from build123d import *

# Parameters (mm, degrees)
BOSS_EXTRUDE1_DEPTH      = 31.75
BOSS_EXTRUDE1_DEPTH_BACK = 31.75
CUT_EXTRUDE2_DEPTH       = 76.011139841
SKETCH3_W                = 3.175
SKETCH3_H                = 76.2
CUT_EXTRUDE3_DEPTH       = 91.870466503


with BuildPart() as part:
    # Sketch1 → Boss-Extrude1 (new body, two sides)
    with BuildSketch(Plane(origin=(0, 0, 0), x_dir=(0, 0, -1), z_dir=(1, 0, 0))) as boss_extrude1_sk:
        with BuildLine():
            Line((1.021340573, 1065.671760022), (10.69404187, 1079.103015809))
            ThreePointArc((10.69404187, 1079.103015809), (11.573445276, 1080.842426323), (11.876332412, 1082.767824636))
            Line((11.876332412, 1082.767824636), (11.876332412, 1187.719530026))
            Line((11.876332412, 1187.719530026), (-13.536061703, 1215.286446683))
            Line((-13.536061703, 1215.286446683), (-19.823769094, 1336.738131825))
            Line((-19.823769094, 1336.738131825), (-36.668668575, 1336.738131825))
            Line((-36.668668575, 1336.738131825), (-41.611308298, 1332.181789519))
            Line((-41.611308298, 1332.181789519), (-19.823769313, 820.101609747))
            ThreePointArc((-19.823769313, 820.101609747), (-14.269049163, 657.404177816), (-11.609546724, 494.633675821))
            ThreePointArc((-11.609546724, 494.633675821), (-11.552697494, 390.848511752), (-12.926889154, 287.072430162))
            ThreePointArc((-12.926889154, 287.072430162), (-14.08497073, 249.282151425), (-16.036320575, 211.524522345))
            ThreePointArc((-16.036320575, 211.524522345), (-18.862629391, 134.694563635), (-17.789412377, 57.820128469))
            ThreePointArc((-17.789412377, 57.820128469), (-14.713555739, 31.224003963), (-7.655684583, 5.397637832))
            ThreePointArc((-7.655684583, 5.397637832), (0, 0), (7.655684583, 5.397637832))
            ThreePointArc((7.655684583, 5.397637832), (14.877278089, 28.754462777), (20.079353087, 52.642348827))
            ThreePointArc((20.079353087, 52.642348827), (27.352586181, 104.395526294), (31.292623673, 156.508551558))
            ThreePointArc((31.292623673, 156.508551558), (31.58109291, 163.474292498), (31.841795924, 170.441127883))
            ThreePointArc((31.841795924, 170.441127883), (33.322524829, 278.033900996), (30.144822487, 385.589931009))
            ThreePointArc((30.144822487, 385.589931009), (12.959303763, 715.76096893), (-4.76677265, 1045.903426895))
            ThreePointArc((-4.76677265, 1045.903426895), (-3.565814336, 1056.283327954), (1.021340573, 1065.671760022))
        make_face()
    extrude(amount=BOSS_EXTRUDE1_DEPTH)
    extrude(boss_extrude1_sk.sketch, amount=-BOSS_EXTRUDE1_DEPTH_BACK)

    # Sketch2 → Cut-Extrude2 (cut, through all)
    with BuildSketch(Plane.XY.offset(-33.399831543)):
        with BuildLine():
            Line((3.96875, 1336.738131825), (19.05, 293.18430056))
            ThreePointArc((19.05, 293.18430056), (18.724333894, 153.044911462), (13.698146022, 12.995306427))
            ThreePointArc((13.698146022, 12.995306427), (9.440831446, 3.765721828), (0, 0))
            Line((0, 0), (31.75, 0))
            Line((31.75, 0), (31.75, 1336.738131825))
            Line((31.75, 1336.738131825), (3.96875, 1336.738131825))
        make_face()
        with BuildLine():
            Line((-31.75, 0), (0, 0))
            ThreePointArc((0, 0), (-9.440831446, 3.765721828), (-13.698146022, 12.995306427))
            ThreePointArc((-13.698146022, 12.995306427), (-18.724333894, 153.044911462), (-19.05, 293.18430056))
            Line((-19.05, 293.18430056), (-3.96875, 1336.738131825))
            Line((-3.96875, 1336.738131825), (-31.75, 1336.738131825))
            Line((-31.75, 1336.738131825), (-31.75, 0))
        make_face()
    extrude(amount=CUT_EXTRUDE2_DEPTH, mode=Mode.SUBTRACT)

    # Sketch3 → Cut-Extrude3 (cut, through all)
    with BuildSketch(Plane(origin=(0, 2.549675539, -49.248855197), x_dir=(-1, 0, 0), z_dir=(0, 0.051702024, -0.998662556))):
        with Locations((0, 1298.746163787)):
            Rectangle(SKETCH3_W, SKETCH3_H)
    extrude(amount=-CUT_EXTRUDE3_DEPTH, mode=Mode.SUBTRACT)


solid = part.part
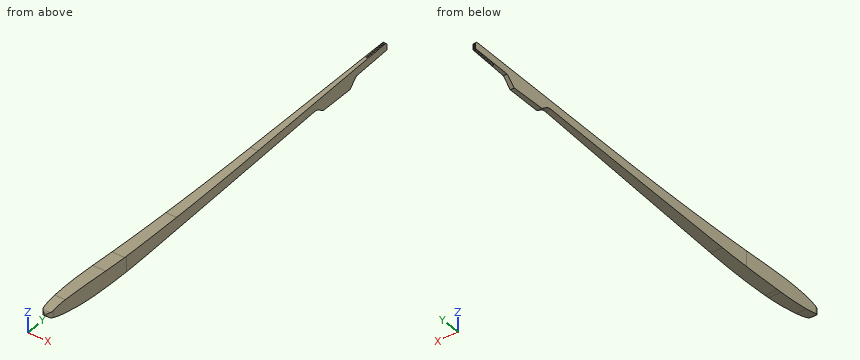
Verification items for the finished model (mm, model axes). Coordinates: 2 decimals unless noted, no trailing zeros. Order: outer loops, then holes, each group sorted by start corner. A loop starts at its lowest first (then second) coordinate and runs counter-clockwise, first axis right, second up. Notation, with made-up numbers: (52.25, 34.25) -> (79.25, 34.25) arc R26 ccw to (79.25, 48.25) -> close; hole circle Ø2 at (-19.75, -24). An arc over 180 degrees is marked (long way). Use CSV: the item, a comma, the result in double quotes. Start each with the question number.
Q1. Section check B-B, the plane y = 713.5. Record the cut outline in (x, z), and give its area (3 significant figures).
Q2. Thickness scan on line 1 along X through (y, z) = (201.5, -28); line 2 along X through (y, z) = (646, -3.5); line 3 along Z through (x, y) = (0.5, 54). Record the ranges inside material, lowest first.
Q3. Section check A-A, the plane y = 510. Record the cut outline in (x, z), and give its area (3 significant figures).
Q4. Depth check by flat-ended pin: P1, Ø20.5, axis at y = 1302, z = 28.5, coming from the -X side; P2, Ø7.5, axis at y = 1280.5, z = 24, coming from the +X side; P3, Ø5, axis at x = -6.5, y = 248.5, coming from the +Z side. Enter the tip coordinate at first touch or a pass-through.
Returned:
1,outline,"(-12.98, -13.08) -> (12.98, -13.08) -> (12.98, 15.86) -> (-12.98, 15.86) -> close"
1,area,"751 mm^2"
2,line 1,"x = -19.37 to 19.37"
2,line 2,"x = -13.95 to 13.95"
2,line 3,"z = -20.31 to 17.6"
3,outline,"(-15.92, -23.73) -> (15.92, -23.73) -> (15.92, 11.74) -> (-15.92, 11.74) -> close"
3,area,"1,130 mm^2"
4,P1,"stops at x = -4.62"
4,P2,"stops at x = 4.84"
4,P3,"stops at z = 14.22"
